Check sheet for the modelled part. Datum: model origin and axes. Units: mm. Round coordinates to 2 decimals unless told otherwise and drop trailing zeros. Loops run counter-clockwise (first coordinate to the right, second up) from the corner with the lowest first, then second, coordinate; pieces in that order, holes last. Notation, with made-up numbers: (24, 45.25) - (58, 45.25) arc R31 ccw to (58, 74.25) - close; hole circle Ø3 at (7.5, 65.5). An arc over 180 degrees is marked (long way). Put each result on its own line as item: value.
```python
from build123d import *

# Parameters (mm, degrees)
ESBO_O1_R                = 6
RESSALTO_EXTRUS_O1_DEPTH = 60
ESBO_O3_R                = 2
CORTE_EXTRUS_O1_DEPTH    = 67.381473319


with BuildPart() as part:
    # Esboço1 → Ressalto-extrusão1 (new body)
    with BuildSketch(Plane.XY):
        with BuildLine():
            Line((-12.5, 0), (-12.5, 13))
            Line((-12.5, 13), (12.5, 13))
            Line((12.5, 13), (12.5, 0))
            ThreePointArc((12.5, 0), (0, -12.5), (-12.5, 0))
        make_face()
        Circle(ESBO_O1_R, mode=Mode.SUBTRACT)
    extrude(amount=RESSALTO_EXTRUS_O1_DEPTH)

    # Esboço3 → Corte-extrusão1 (cut, through all)
    with BuildSketch(Plane(origin=(0, 13, 0), x_dir=(1, 0, 0), z_dir=(0, 1, 0))):
        with Locations(Location((-9, -52.5, 0), (0, 0, 270))):
            Circle(ESBO_O3_R)
        with Locations(Location((-9, -7.5, 0), (0, 0, 270))):
            Circle(ESBO_O3_R)
        with Locations(Location((9, -52.5, 0), (0, 0, 270))):
            Circle(ESBO_O3_R)
        with Locations(Location((9, -7.5, 0), (0, 0, 270))):
            Circle(ESBO_O3_R)
    extrude(amount=-CORTE_EXTRUS_O1_DEPTH, mode=Mode.SUBTRACT)


solid = part.part
```
Item 1: Section check C-C on z = 52.5. Enter the section's corners in (x, y), then the cut area to 3 significant figures.
Filled sheet:
outline: (-12.5, 0) arc R12.5 ccw to (-11, -5.94) - (-11, 13) - (-12.5, 13) - close; (-7, -10.36) arc R12.5 ccw to (7, -10.36) - (7, 13) - (-7, 13) - close; (11, -5.94) arc R12.5 ccw to (12.5, 0) - (12.5, 13) - (11, 13) - close; hole circle Ø12 at (0, 0)
area: 285 mm²
Item 2: Section check D-D on y = 3.5. Enter the section's corners in (x, z).
Filled sheet:
outline: (-12.5, 0) - (-4.87, 0) - (-4.87, 60) - (-12.5, 60) - close; (4.87, 0) - (12.5, 0) - (12.5, 60) - (4.87, 60) - close; hole circle Ø4 at (-9, 7.5); hole circle Ø4 at (-9, 52.5); hole circle Ø4 at (9, 7.5); hole circle Ø4 at (9, 52.5)
Item 3: Release check for a two-part mould opening along Z. For faces 1 (the cylindrical face through (7.226, 1.485, 53.423)), 2 (the flat face through (0, 13, 30)), 3 (the cylindrical face through (-7.017, 1.485, 7.24)), 4 (the flat face through (3, 6, 0)) record: +Z half, -Z half, draft (parallel to the pull), parting line (faces both ways), or undercut.
Filled sheet:
face 1: undercut
face 2: draft
face 3: undercut
face 4: -Z half
Item 4: Section check B-B on y = 6.75. Enter the section's corners in (x, z), then the cut area to 3 significant figures.
Filled sheet:
outline: (-12.5, 0) - (12.5, 0) - (12.5, 60) - (-12.5, 60) - close; hole circle Ø4 at (-9, 7.5); hole circle Ø4 at (-9, 52.5); hole circle Ø4 at (9, 7.5); hole circle Ø4 at (9, 52.5)
area: 1,450 mm²
Item 5: Section check A-A on x = 0. Enter the section's corners in (y, z), then the cut area to 3 significant figures.
Filled sheet:
outline: (-12.5, 0) - (-6, 0) - (-6, 60) - (-12.5, 60) - close; (6, 0) - (13, 0) - (13, 60) - (6, 60) - close
area: 810 mm²
Item 6: Go/stop test with flat-tipped pins: pin 1 (2.5 mm diameter, centred on x = 9, z = 7.5, fed in from -Y); pin 2 (3 mm diameter, centred on x = 6, z = 31.5, fed in from -Y); pin 3 (12 mm diameter, centred on y = -10, z = 25.5, fed in from +X); pin 4 (4.5 mm diameter, centred on x = -9, z = 52.5, fed in from -Y). Record where each tip stops, or that it passes through.
Filled sheet:
pin 1: through
pin 2: y = -11.66
pin 3: x = 11.84
pin 4: y = -10.52
Item 7: Thickness scan on line 1 (Z direction, x = -9, y = 7.75); line 2 (X direction, y = -3, z = 7.5); line 3 (Z direction, x = 9.5, y = -3). Record the ranges inside material, lowest first. Write a range as from..to.
Filled sheet:
line 1: 0..5.5, 9.5..50.5, 54.5..60
line 2: -12.13..-11, -7..-5.2, 5.2..7, 11..12.13
line 3: 0..5.56, 9.44..50.56, 54.44..60
